from build123d import *

# Parameters (mm, degrees)
ESQUISSE1_W      = 9.5
ESQUISSE1_H      = 9.5
EXTRUSION1_DEPTH = 3.2
ESQUISSE2_R      = 1.5
EXTRUSION2_DEPTH = 3
ESQUISSE3_R      = 1.8
EXTRUSION3_DEPTH = 5
EXTRUSION3_TAPER = 6
ESQUISSE4_R      = 1.9
EXTRUSION4_DEPTH = 4
ESQUISSE5_R      = 2.2
EXTRUSION5_DEPTH = 5
EXTRUSION5_TAPER = 7


with BuildPart() as part:
    # Esquisse1 → Extrusion1 (new body)
    with BuildSketch(Plane.XY):
        with Locations((-2.457587253, -3.276631259)):
            Rectangle(ESQUISSE1_W, ESQUISSE1_H)
    extrude(amount=EXTRUSION1_DEPTH)

    # Esquisse2 → Extrusion2 (add)
    with BuildSketch(Plane.XY.offset(3.2)):
        with Locations((-2.457587253, -3.276631259)):
            Circle(ESQUISSE2_R)
    extrude(amount=EXTRUSION2_DEPTH)

    # Esquisse3 → Extrusion3 (add)
    with BuildSketch(Plane.XY.offset(6.2)):
        with Locations((-2.457587253, -3.276631259)):
            Circle(ESQUISSE3_R)
    extrude(amount=EXTRUSION3_DEPTH, taper=EXTRUSION3_TAPER)

    # Esquisse4 → Extrusion4 (add)
    with BuildSketch(Plane(origin=(0, 0, 0), x_dir=(-1, 0, 0), z_dir=(0, 0, -1))):
        with Locations(Location((2.457587253, -3.276631259, 0), (0, 0, 180))):
            Circle(ESQUISSE4_R)
    extrude(amount=EXTRUSION4_DEPTH)

    # Esquisse5 → Extrusion5 (add)
    with BuildSketch(Plane(origin=(0, 0, -4), x_dir=(-1, 0, 0), z_dir=(0, 0, -1))):
        with Locations((2.457587253, -3.276631259)):
            Circle(ESQUISSE5_R)
    extrude(amount=EXTRUSION5_DEPTH, taper=EXTRUSION5_TAPER)


solid = part.part
Work out the finished part from the listing and answer in its coordinate system (mm). Coordinates: 2 decimals unless noted, no trailing zeros. Write each loop counter-clockwise with the first axis right and the second up, starting at its lowest first coordinate (ties: lowest second). Pieces come first, ordered by that corner, then holes. Notation, with made-up numbers: M 16,65 L 28,65 A30 ccw 28,103 Z; hole C 57,-23.75 d6. An arc over 180 degrees is marked long. Answer as CSV lines item,"result". Start each with the question number.
Item 1: Section B-B on z = -3.5 is taken. Write down the section's boundary in (x, y).
Item 2: Section A-A on x = 0 is taken. Write down the section's boundary in (y, z).
Item 3: Consider L1, parallel to Z at x = 0.75, y = 1; L2, parallel to Y at x = -1.5, z = 10.25; L3, parallel to X at y = -3.75, z = 9.5. Determine where each line is inside the solid, lowest interval first.
Item 4: Section D-D on z = 6.5 is taken. Write down the section's boundary in (x, y).
Item 5: Determine the mould class of faces 1 (the face through (-3, 1.473, 2)), 2 (the face through (-2.78, -4.74, 4.68)), 3 (the face through (-3.965, -2.121, -1.972)), 4 (the face through (-2.79, -4.774, 8.735)) for opening direction Z: released by +Z, released by -Z, zero draft, split by the parting line, or undercut.
Item 6: Flat-ended cylindrical pins translate along their axes: P1, Ø3, axis at x = 1, z = -4, coming from the +Y side; P2, Ø2, axis at x = -1.5, z = -2, coming from the -Y side; P3, Ø3, axis at x = 0, z = 9, coming from the -Y side. Find the tip coordinate at first contact, or state that the pin passes through.
Item 7: Section C-C on y = -6.5 is taken. Write down the section's boundary in (x, z).
Checks:
1,outline,"C -2.46,-3.28 d3.8"
2,outline,"M -8.03,0 L 1.47,0 L 1.47,3.2 L -8.03,3.2 Z"
3,L1,"z = 0 to 3.2"
3,L2,"y = -4.26 to -2.29"
3,L3,"x = -3.83 to -1.08"
4,outline,"C -2.46,-3.28 d3.54"
5,face 1,"zero draft"
5,face 2,"undercut"
5,face 3,"undercut"
5,face 4,"released by +Z"
6,P1,"stops at y = -2.27"
6,P2,"stops at y = -5.18"
6,P3,"stops at y = -4.46"
7,outline,"M -7.21,0 L 2.29,0 L 2.29,3.2 L -7.21,3.2 Z"
